For this review, take the finished solid that the model builds, in its own axes (mm). A direction names the side the tool comes from. Round coordinates to 2 decimals unless told otherwise and drop trailing zeros. Write each loop counter-clockwise with the first axis right and the second up, starting at its lowest first coordinate (ties: lowest second). Pieces come first, ordered by that corner, then holes. Notation, with made-up numbers: M 64.5,79 L 92.5,79 A36 ccw 92.5,118 Z; hole C 86,77.5 d4. An arc over 180 degrees is marked long. Answer in a Markdown table with one row per item.
```python
from build123d import *

# Parameters (mm, degrees)
SKETCH3_W                                       = 57.15
SKETCH3_H                                       = 50
BOSS_EXTRUDE1_DEPTH                             = 8
SKETCH3_3_R                                     = 1.5
SKETCH3_3_R_2                                   = 8
CUT_EXTRUDE2_DEPTH                              = 10
SKETCH4_R                                       = 18.5
CUT_EXTRUDE3_DEPTH                              = 4
BOSS_EXTRUDE2_DEPTH                             = 15
BOSS_EXTRUDE2_DEPTH_BACK                        = 23
SKETCH6_W                                       = 101.6
SKETCH6_H                                       = 5
CSK_FOR_M3_FLAT_HEAD_MACHINE_SCREW1_D           = 3.4
CSK_FOR_M3_FLAT_HEAD_MACHINE_SCREW1_CSINK_D     = 6.3
CSK_FOR_M3_FLAT_HEAD_MACHINE_SCREW1_CSINK_ANGLE = 90
CUT_EXTRUDE6_REACH                              = 555.432
SKETCH16_R                                      = 1.7
CUT_EXTRUDE7_REACH                              = 73.656
SKETCH17_W                                      = 25.08228791
SKETCH17_H                                      = 11.980848154
SKETCH18_W                                      = 17.78
SKETCH18_H                                      = 8
BOSS_EXTRUDE3_DEPTH                             = 45
SKETCH13_R                                      = 6.7056
SKETCH13_R_2                                    = 4.8006
BOSS_EXTRUDE4_DEPTH                             = 5.08
CUT_EXTRUDE8_START                              = -5.08
SKETCH19_R                                      = 4.8006
CUT_EXTRUDE8_DEPTH                              = 5.08
BOSS_EXTRUDE5_DEPTH                             = 2.54


with BuildPart() as part:
    # Sketch3 → Boss-Extrude1 (new body)
    with BuildSketch(Plane.XY):
        with Locations((0, 25)):
            Rectangle(SKETCH3_W, SKETCH3_H)
    extrude(amount=BOSS_EXTRUDE1_DEPTH)

    # Sketch3<3> → Cut-Extrude2 (cut)
    with BuildSketch(Plane.XY):
        with Locations(Location((-7.75, 38.423393759, 0), (0, 0, 180))):
            Circle(SKETCH3_3_R)
        with Locations(Location((7.75, 38.423393759, 0), (0, 0, 180))):
            Circle(SKETCH3_3_R)
        with Locations(Location((-7.75, 11.576606241, 0), (0, 0, 180))):
            Circle(SKETCH3_3_R)
        with Locations(Location((7.75, 11.576606241, 0), (0, 0, 180))):
            Circle(SKETCH3_3_R)
        with Locations(Location((15.5, 25, 0), (0, 0, 180))):
            Circle(SKETCH3_3_R)
        with Locations(Location((6.062177825, 28.499999999, 0), (0, 0, 180))):
            Circle(SKETCH3_3_R_2)
    extrude(amount=CUT_EXTRUDE2_DEPTH, mode=Mode.SUBTRACT)

    # Sketch4 → Cut-Extrude3 (cut)
    with BuildSketch(Plane.XY.offset(8)):
        with Locations((0, 25)):
            Circle(SKETCH4_R)
    extrude(amount=-CUT_EXTRUDE3_DEPTH, mode=Mode.SUBTRACT)

    # Sketch6 → Boss-Extrude2 (add, two sides: drawn at the far end of the back side and taken through both)
    with BuildSketch(Plane.XY.offset(8).offset(-BOSS_EXTRUDE2_DEPTH_BACK)):
        with Locations((0, 2.5)):
            Rectangle(SKETCH6_W, SKETCH6_H)
    extrude(amount=BOSS_EXTRUDE2_DEPTH + BOSS_EXTRUDE2_DEPTH_BACK)

    # CSK for M3 Flat Head Machine Screw1 (through all)
    with Locations(Plane(origin=(0, 5, 0), x_dir=(1, 0, 0), z_dir=(0, 1, 0))):
        with Locations((-43.3, 7.5), (-43.3, -15.5), (43.3, -15.5), (43.3, 7.5)):
            CounterSinkHole(CSK_FOR_M3_FLAT_HEAD_MACHINE_SCREW1_D / 2, CSK_FOR_M3_FLAT_HEAD_MACHINE_SCREW1_CSINK_D / 2, counter_sink_angle=CSK_FOR_M3_FLAT_HEAD_MACHINE_SCREW1_CSINK_ANGLE)

    # Sketch16 → Cut-Extrude6 (cut, up to next)
    with BuildSketch(Plane(origin=(-499.248949842, 16.821159134, -28.308871479), x_dir=(0.050830850863696445, -0.0009181581696577921, 0.9987068546806156), z_dir=(0.036090886531912156, 0.9993480899541041, -0.0009181581696584951)), mode=Mode.PRIVATE) as cut_extrude6_sk1:
        with Locations((67.5, 464.499999998)):
            Circle(SKETCH16_R)
    cut_extrude6_tool1 = extrude(cut_extrude6_sk1.sketch, amount=-CUT_EXTRUDE6_REACH, mode=Mode.PRIVATE) & part.part
    # Sketch16 → Cut-Extrude6 (cut, up to next)
    with BuildSketch(Plane(origin=(-499.248949842, 16.821159134, -28.308871479), x_dir=(0.050830850863696445, -0.0009181581696577921, 0.9987068546806156), z_dir=(0.036090886531912156, 0.9993480899541041, -0.0009181581696584951)), mode=Mode.PRIVATE) as cut_extrude6_sk2:
        with Locations((44.5, 464.499999998)):
            Circle(SKETCH16_R)
    cut_extrude6_tool2 = extrude(cut_extrude6_sk2.sketch, amount=-CUT_EXTRUDE6_REACH, mode=Mode.PRIVATE) & part.part
    add(cut_extrude6_tool1.solids().sort_by_distance((-32.221346, -0.005033, 15.492911))[0], mode=Mode.SUBTRACT)
    add(cut_extrude6_tool2.solids().sort_by_distance((-33.390455, 0.016084, -7.477347))[0], mode=Mode.SUBTRACT)

    # Sketch17 → Cut-Extrude7 (cut, up to next)
    with BuildSketch(Plane(origin=(0, 5, 0), x_dir=(1, 0, 0), z_dir=(0, 1, 0)), mode=Mode.PRIVATE) as cut_extrude7_sk1:
        with Locations((-38.258856045, 9.009575923)):
            Rectangle(SKETCH17_W, SKETCH17_H)
    cut_extrude7_tool1 = extrude(cut_extrude7_sk1.sketch, amount=-CUT_EXTRUDE7_REACH, mode=Mode.PRIVATE) & part.part
    add(cut_extrude7_tool1.solids().sort_by_distance((-38.258856, 5, -9.009576))[0], mode=Mode.SUBTRACT)

    # Sketch18 → Boss-Extrude3 (add)
    with BuildSketch(Plane(origin=(0, 5, 0), x_dir=(1, 0, 0), z_dir=(0, 1, 0))):
        with Locations((-37.465, -4)):
            Rectangle(SKETCH18_W, SKETCH18_H)
    extrude(amount=BOSS_EXTRUDE3_DEPTH)

    # Sketch13 → Boss-Extrude4 (add)
    with BuildSketch(Plane(origin=(0, 0, 0), x_dir=(-1, 0, 0), z_dir=(0, 0, -1))):
        with Locations((38.117822207, 28.499999999)):
            Circle(SKETCH13_R)
        with Locations((38.117822207, 28.499999999)):
            Circle(SKETCH13_R_2, mode=Mode.SUBTRACT)
    extrude(amount=BOSS_EXTRUDE4_DEPTH)

    # Sketch19 → Cut-Extrude8 (cut)
    with BuildSketch(Plane(origin=(0, 0, 0), x_dir=(-1, 0, 0), z_dir=(0, 0, -1)).offset(CUT_EXTRUDE8_START)):
        with Locations((38.117822207, 28.499999999)):
            Circle(SKETCH19_R)
    extrude(amount=CUT_EXTRUDE8_DEPTH, mode=Mode.SUBTRACT)

    # Sketch20 → Boss-Extrude5 (add)
    with BuildSketch(Plane.XZ):
        Polygon((-50.8, -3.019151846), (-50.8, 23), (50.8, 23), (50.8, -15), (-25.71771209, -15), (-25.71771209, -3.019151846), align=None)
    extrude(amount=BOSS_EXTRUDE5_DEPTH)


solid = part.part
```
Q1. Take a section at A-A (x = 7.75). State the section outline as (y, z) points.
Found:
| item | result |
|---|---|
| outline | M -2.54,-15 L 5,-15 L 5,0 L 10.08,0 L 10.08,4 L 8.2,4 L 8.2,8 L 5,8 L 5,23 L -2.54,23 Z; M 13.08,0 L 20.68,0 L 20.68,4 L 13.08,4 Z; M 36.32,0 L 36.92,0 L 36.92,4 L 36.32,4 Z; M 39.92,0 L 50,0 L 50,8 L 41.8,8 L 41.8,4 L 39.92,4 Z |
Q2. For probe 1 along Z at (x, y) = (43.3, 1.95); probe 2 along X at (y, z) = (1.75, 15.5); probe 3 along Y at (x, z) = (-7.75, 2.05), list the stretches that pass through material, from the lowest coordinate up.
Found:
| item | result |
|---|---|
| probe 1 | -15 to -9.2, -5.8 to 13.8, 17.2 to 23 |
| probe 2 | -50.8 to -45, -41.6 to 41.6, 45 to 50.8 |
| probe 3 | -2.54 to 10.08, 13.08 to 36.92, 39.92 to 50 |
Q3. Take a section at C-C (x = 23). State the section outline as (y, z) points.
Found:
| item | result |
|---|---|
| outline | M -2.54,-15 L 5,-15 L 5,0 L 50,0 L 50,8 L 5,8 L 5,23 L -2.54,23 Z |
Q4. Insertion check: P1, Ø3, axis at y = 39.5, z = 6, coming from the -X side (3 decimals); P2, Ø4.5, axis at x = 43.3, z = -7.5, coming from the +Y side; P3, Ø6.5, axis at x = -39.5, y = 29, coming from the -Z side. Each pin has a flat end and moves straight along its axis. Give the tip position at first contact, or say it passes through.
Found:
| item | result |
|---|---|
| P1 | x = -46.355 |
| P2 | y = 4.1 |
| P3 | z = 5.08 |
Q5. Take a section at B-B (y = 28.5). State the section outline as (x, z) points (3 decimals), then the cut area to 3 significant figures.
Found:
| item | result |
|---|---|
| outline | M -46.355,0 L -44.823,0 L -44.823,-5.08 L -42.918,-5.08 L -42.918,5.08 L -33.317,5.08 L -33.317,-5.08 L -31.412,-5.08 L -31.412,0 L -1.938,0 L -1.938,4 L -18.166,4 L -18.166,8 L -46.355,8 Z; M 14.062,0 L 28.575,0 L 28.575,8 L 18.166,8 L 18.166,4 L 14.062,4 Z |
| area | 361 mm² |
Q6. Take a section at D-D (z = -7.5). State the section outline as (x, y) points.
Found:
| item | result |
|---|---|
| outline | M -25.72,-2.54 L 50.8,-2.54 L 50.8,5 L 46.45,5 L 45,3.55 L 45,0 L 41.6,0 L 41.6,3.55 L 40.15,5 L -25.72,5 Z |
Q7. Machinability: for faces 1 (the face through (-18, 32, 8)), 2 (the face through (28.575, 27, 4)), 3 (the face through (-43, 0, 16)), which of the approach directions +Z, -Z, +X, -X, +Y, -Y give a long, thin tool a straight path to every point of the face, cutting with its end or side? Answer none if there is none.
Found:
| item | result |
|---|---|
| face 1 | +Z, +X, -X, +Y |
| face 2 | +Z, -Z, +X, +Y |
| face 3 | +Y |
Q8. Mouldability with a two-part tool opening along Y and no side actions: class faces 4 (the face through (-44.92, 1.75, 14.99)), 5 (the face through (-9, 50, 4)), 6 (the face through (-6.644, 10.563, 1.972)) as +Y half, -Y half, draft (parallel to the pull), parting line (faces both ways), or undercut.
Found:
| item | result |
|---|---|
| face 4 | draft |
| face 5 | +Y half |
| face 6 | undercut |
